Read the model definition and answer for the solid it produces. Units are mm, in the model's axes. A direction names the side the tool comes from. Round coordinates to 2 decimals unless told otherwise and drop trailing zeros. Order: outer loops, then holes, each group sorted by start corner. A loop starts at its lowest first (then second) coordinate and runs counter-clockwise, first axis right, second up.
from build123d import *

# Parameters (mm, degrees)
F1_DEPTH = 80
F2_R     = 10
F3_DEPTH = 20


with BuildPart() as f1:
    # F0 (on Front) → F1 (new body)
    with BuildSketch(Plane.XZ):
        Polygon((0, 20), (0, 0), (60, 0), (60, 20), (40, 20), (40, 10), (20, 10), (20, 20), align=None)
    extrude(amount=-F1_DEPTH)

    # F2 (on face) → F3 (cut)
    with BuildSketch(Plane(origin=(0, 0, 0), x_dir=(1, 0, 0), z_dir=(0, 0, -1))):
        with Locations((30, -40)):
            Circle(F2_R)
    extrude(amount=-F3_DEPTH, mode=Mode.SUBTRACT)


solid = f1.part
Q1. A cutting plane is placed at A-A, the plane z = 15. Give the vertices of the cut face in (x, y), plus the area to 3 significant figures.
Outcome:
outline: (0, 0) - (20, 0) - (20, 80) - (0, 80) - close; (40, 0) - (60, 0) - (60, 80) - (40, 80) - close
area: 3,200 mm2
Q2. A flat-ended cylindrical pin translates along its axis: pin 1 (6 mm diameter, centred on x = 25, y = 56, fed in from +Z). Find the tip coordinate at first contact, or state that the pin passes through.
Outcome:
pin 1: stops at z = 10
Q3. A cutting plane is placed at C-C, the plane z = 2.5. Give the vertices of the cut face in (x, y), plus the area to 3 significant figures.
Outcome:
outline: (0, 0) - (60, 0) - (60, 80) - (0, 80) - close; hole circle Ø20 at (30, 40)
area: 4,490 mm2
Q4. Straight lines are drawn through the part: probe 1 along X at (y, z) = (40, 6.5); probe 2 along Y at (x, z) = (30, 3); probe 3 along Z at (x, y) = (36.5, 52). For each, find the intervals that lie inside material, in ascending order.
Outcome:
probe 1: x = 0 to 20, 40 to 60
probe 2: y = 0 to 30, 50 to 80
probe 3: z = 0 to 10
Q5. For a pull along X with two mould halves and no side action, classify faces 1 (the face through (30, 15, 10)), 2 (the face through (60, 39, 10)), 3 (the face through (40, 39, 15)), 4 (the face through (50, 39, 20)) as released by +X, released by -X, zero draft, split by the parting line, or undercut.
Outcome:
face 1: undercut
face 2: released by +X
face 3: undercut
face 4: zero draft
Q6. A cutting plane is placed at B-B, the plane x = 30. Give the vertices of the cut face in (y, z).
Outcome:
outline: (0, 0) - (30, 0) - (30, 10) - (0, 10) - close; (50, 0) - (80, 0) - (80, 10) - (50, 10) - close
Q7. A cutting plane is placed at D-D, the plane y = 13. Give the vertices of the cut face in (x, z), plus the area to 3 significant figures.
Outcome:
outline: (0, 0) - (60, 0) - (60, 20) - (40, 20) - (40, 10) - (20, 10) - (20, 20) - (0, 20) - close
area: 1,000 mm2
Q8. For faces 5 (the face through (20, 39, 15)), 6 (the face through (23, 31, 0)), determine the directions among +Z, -Z, +X, -X, +Y, -Y from which every point of the face is accessible in a straight line to the end or side of a thin tool.
Outcome:
face 5: +Z, +Y, -Y
face 6: -Z, +X, -X, +Y, -Y
